```python
from build123d import *

# Parameters (mm, degrees)
BOSS_EXTRUDE1_DEPTH = 5
CUT_EXTRUDE1_REACH  = 7
SKETCH2_W           = 8
SKETCH2_H           = 5.2
CUT_EXTRUDE2_DEPTH  = 5
CUT_EXTRUDE3_REACH  = 7
SKETCH5_R           = 1


with BuildPart() as part:
    # Sketch1 → Boss-Extrude1 (new body)
    with BuildSketch(Plane.XY):
        with BuildLine():
            Line((24.485627442, 0), (69.985627442, 0))
            Line((69.985627442, 0), (69.985627442, 20))
            Line((69.985627442, 20), (-15.014372558, 20))
            Line((-15.014372558, 20), (-15.014372558, 0))
            Line((-15.014372558, 0), (-2.514372558, 0))
            ThreePointArc((-2.514372558, 0), (1.021161348, -1.464466094), (2.485627442, -5))
            Line((2.485627442, -5), (2.485627442, -10.5))
            ThreePointArc((2.485627442, -10.5), (3.217860489, -12.267766953), (4.985627442, -13))
            Line((4.985627442, -13), (16.528766582, -13))
            ThreePointArc((16.528766582, -13), (18.58372754, -12.464616991), (19.485627442, -10.542098831))
            Line((19.485627442, -10.542098831), (19.485627442, -5))
            ThreePointArc((19.485627442, -5), (20.950093536, -1.464466094), (24.485627442, 0))
        make_face()
    extrude(amount=BOSS_EXTRUDE1_DEPTH)

    # Sketch2 → Cut-Extrude1 (cut, up to next)
    with BuildSketch(Plane.XY.offset(5), mode=Mode.PRIVATE) as cut_extrude1_sk1:
        with Locations((-1.014372558, 4.6)):
            Rectangle(SKETCH2_W, SKETCH2_H)
    cut_extrude1_tool1 = extrude(cut_extrude1_sk1.sketch, amount=-CUT_EXTRUDE1_REACH, mode=Mode.PRIVATE) & part.part
    add(cut_extrude1_tool1.solids().sort_by_distance((-1.014373, 4.6, 5))[0], mode=Mode.SUBTRACT)
    # Sketch2 → Cut-Extrude1 (cut, up to next)
    with BuildSketch(Plane.XY.offset(5), mode=Mode.PRIVATE) as cut_extrude1_sk2:
        with Locations((17.985627442, 4.6)):
            Rectangle(SKETCH2_W, SKETCH2_H)
    cut_extrude1_tool2 = extrude(cut_extrude1_sk2.sketch, amount=-CUT_EXTRUDE1_REACH, mode=Mode.PRIVATE) & part.part
    add(cut_extrude1_tool2.solids().sort_by_distance((17.985627, 4.6, 5))[0], mode=Mode.SUBTRACT)
    # Sketch2 → Cut-Extrude1 (cut, up to next)
    with BuildSketch(Plane.XY.offset(5), mode=Mode.PRIVATE) as cut_extrude1_sk3:
        with Locations((36.985627442, 4.6)):
            Rectangle(SKETCH2_W, SKETCH2_H)
    cut_extrude1_tool3 = extrude(cut_extrude1_sk3.sketch, amount=-CUT_EXTRUDE1_REACH, mode=Mode.PRIVATE) & part.part
    add(cut_extrude1_tool3.solids().sort_by_distance((36.985627, 4.6, 5))[0], mode=Mode.SUBTRACT)
    # Sketch2 → Cut-Extrude1 (cut, up to next)
    with BuildSketch(Plane.XY.offset(5), mode=Mode.PRIVATE) as cut_extrude1_sk4:
        with Locations((55.985627442, 4.6)):
            Rectangle(SKETCH2_W, SKETCH2_H)
    cut_extrude1_tool4 = extrude(cut_extrude1_sk4.sketch, amount=-CUT_EXTRUDE1_REACH, mode=Mode.PRIVATE) & part.part
    add(cut_extrude1_tool4.solids().sort_by_distance((55.985627, 4.6, 5))[0], mode=Mode.SUBTRACT)

    # Sketch3 → Cut-Extrude2 (cut)
    with BuildSketch(Plane.XY.offset(5)):
        with BuildLine():
            Line((-9.514372558, 20), (0.485627442, 20))
            Line((0.485627442, 20), (0.485627442, 15.5))
            ThreePointArc((0.485627442, 15.5), (-0.393052215, 13.378679656), (-2.514372558, 12.5))
            Line((-2.514372558, 12.5), (-6.514372558, 12.5))
            ThreePointArc((-6.514372558, 12.5), (-8.635692902, 13.378679656), (-9.514372558, 15.5))
            Line((-9.514372558, 15.5), (-9.514372558, 20))
        make_face()
    cut_extrude2 = extrude(amount=-CUT_EXTRUDE2_DEPTH, mode=Mode.SUBTRACT)

    # Mirror1: Cut-Extrude2 across plane
    add(cut_extrude2.mirror(Plane(origin=(27.485627442, 0, 0), x_dir=(0, 0, 1), z_dir=(1, 0, 0))), mode=Mode.SUBTRACT)

    # Sketch5 → Cut-Extrude3 (cut, up to next)
    with BuildSketch(Plane.XY.offset(5), mode=Mode.PRIVATE) as cut_extrude3_sk1:
        with Locations((6.235627442, 9)):
            Circle(SKETCH5_R)
    cut_extrude3_tool1 = extrude(cut_extrude3_sk1.sketch, amount=-CUT_EXTRUDE3_REACH, mode=Mode.PRIVATE) & part.part
    add(cut_extrude3_tool1.solids().sort_by_distance((6.235627, 9, 5))[0], mode=Mode.SUBTRACT)
    # Sketch5 → Cut-Extrude3 (cut, up to next)
    with BuildSketch(Plane.XY.offset(5), mode=Mode.PRIVATE) as cut_extrude3_sk2:
        with Locations((48.735627442, 9)):
            Circle(SKETCH5_R)
    cut_extrude3_tool2 = extrude(cut_extrude3_sk2.sketch, amount=-CUT_EXTRUDE3_REACH, mode=Mode.PRIVATE) & part.part
    add(cut_extrude3_tool2.solids().sort_by_distance((48.735627, 9, 5))[0], mode=Mode.SUBTRACT)
    # Sketch5 → Cut-Extrude3 (cut, up to next)
    with BuildSketch(Plane.XY.offset(5), mode=Mode.PRIVATE) as cut_extrude3_sk3:
        with Locations((6.235627442, -9)):
            Circle(SKETCH5_R)
    cut_extrude3_tool3 = extrude(cut_extrude3_sk3.sketch, amount=-CUT_EXTRUDE3_REACH, mode=Mode.PRIVATE) & part.part
    add(cut_extrude3_tool3.solids().sort_by_distance((6.235627, -9, 5))[0], mode=Mode.SUBTRACT)


solid = part.part
```
For this review, take the finished solid that the model builds, in its own axes (mm). A direction names the side the tool comes from. Give positions to 0.01 mm unless a question says otherwise; leave off trailing zeros. Write each loop counter-clockwise with the first axis right and the second up, starting at its lowest first coordinate (ties: lowest second). Pieces come first, ordered by that corner, then holes. Notation, with made-up numbers: M 29,-31 L 46,-31 A15 cw 46,-16 Z; hole C -16,61.5 d7. An arc over 180 degrees is marked long. Answer as CSV lines item,"result".
1. For faces 1 (the flat face through (56, 7.2, 3)), 2 (the flat face through (47, 0, 2)), 3 (the flat face through (-4, 12.5, 3)), list the 3-axis set-ups (+Z, -Z, +X, -X, +Y, -Y) from which the entire face can be reached by the end or side of a thin tool; tool diameter is ignored.
Findings:
face 1,"+Z, -Z"
face 2,"+Z, -Z, +X, -Y"
face 3,"+Z, -Z, +Y"
2. Consider section B-B, the plane x = 36.5. Write out the cut boundary in (y, z), then the cut area to 3 significant figures.
Findings:
outline,"M 0,0 L 2,0 L 2,5 L 0,5 Z; M 7.2,0 L 20,0 L 20,5 L 7.2,5 Z"
area,"74.0 mm2"
3. Consider section D-D, the plane z = 2.2. Count the separate pieces of the cut face and the enclosed holes in it, then the cut area to 3 significant figures.
Findings:
separate pieces,"1"
enclosed holes,"7"
area,"1,610 mm2"
4. For pin 1 (2.5 mm diameter, centred on x = 0.5, z = 2.5, fed in from -Y); pin 2 (2 mm diameter, centred on x = 59, z = 2, fed in from +Y); pin 3 (2.5 mm diameter, centred on x = 58, z = 1.5, fed in from -Y), all flat-tipped, find the tip position at first contact; note any pin that passes through.
Findings:
pin 1,"stops at y = -2.39"
pin 2,"stops at y = 12.5"
pin 3,"stops at y = 0"
5. Consider section A-A, the plane y = -9. Write out the cut boundary in (x, z), then the cut area to 3 significant figures.
Findings:
outline,"M 2.49,0 L 5.24,0 L 5.24,5 L 2.49,5 Z; M 7.24,0 L 19.49,0 L 19.49,5 L 7.24,5 Z"
area,"75.0 mm2"
6. Draft analysis for pull direction Y (two halves, no side actions). For faces 4 (the flat face through (-1, 7.2, 3)), 5 (the flat face through (-9, 0, 2)), 6 (the cylindrical face through (-8.612, 13.355, 2.535)), state which applies: +Y half, -Y half, draft (parallel to the pull), parting line (faces both ways), or undercut.
Findings:
face 4,"undercut"
face 5,"-Y half"
face 6,"+Y half"
7. Wall thickness on line 1 (X direction, y = 4, z = 3.35); line 2 (Y direction, x = -4, z = 3.75); line 3 (Y direction, x = 15, z = 3.15): over which ranges is each line inside the solid? List them lowest first.
Findings:
line 1,"x = -15.01 to -5.01, 2.99 to 13.99, 21.99 to 32.99, 40.99 to 51.99, 59.99 to 69.99"
line 2,"y = 0 to 2, 7.2 to 12.5"
line 3,"y = -13 to 2, 7.2 to 20"
8. Consider section C-C, the plane y = 9. Write out the cut boundary in (x, z).
Findings:
outline,"M -15.01,0 L 5.24,0 L 5.24,5 L -15.01,5 Z; M 7.24,0 L 47.74,0 L 47.74,5 L 7.24,5 Z; M 49.74,0 L 69.99,0 L 69.99,5 L 49.74,5 Z"
